from build123d import *

# Parameters (mm, degrees)
F0_R     = 36
F1_DEPTH = 125
F2_R     = 12.7
F3_DEPTH = 254
F4_R     = 10.16


with BuildPart() as f1:
    # F0 (on Right) → F1 (new body)
    with BuildSketch(Plane.YZ):
        with Locations((-19.977277, 22.49966)):
            Circle(F0_R)
    extrude(amount=F1_DEPTH)

    # F2 (on face) → F3 (cut)
    with BuildSketch(Plane(origin=(0, 0, 0), x_dir=(0, -1, 0), z_dir=(-1, 0, 0))):
        with Locations((19.977277, 22.49966)):
            Circle(F2_R)
    extrude(amount=-F3_DEPTH, mode=Mode.SUBTRACT)

    # F4
    f4_edges = [f1.edges().sort_by_distance(p)[0] for p in [
        (0, -55.977277, 22.49966),
        (125, -55.977277, 22.49966),
    ]]
    fillet(f4_edges, radius=F4_R)


solid = f1.part
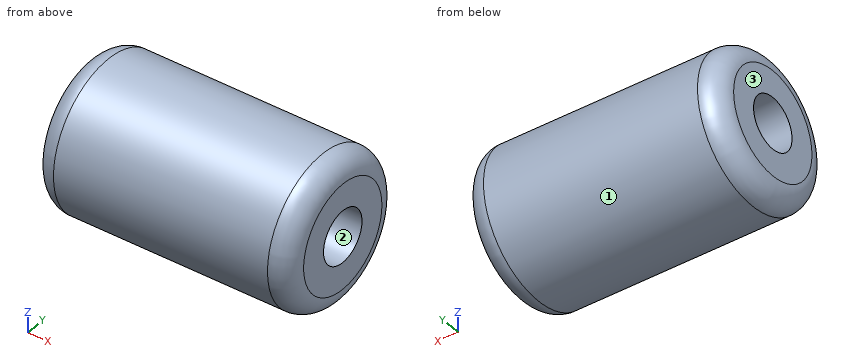
Geometry check sheet. Reference: the model listing, model coordinates, mm. Face numbers are marked on the shaded views. Round coordinates to 2 decimals unless told otherwise and drop trailing zeros. Order: outer loops, then holes, each group sorted by start corner. A loop starts at its lowest first (then second) coordinate and runs counter-clockwise, first axis right, second up. Notation, with made-up numbers: M -14,60.25 L 15,60.25 A34 ccw 15,95.25 Z; hole C 27,40.5 d9. An arc over 180 degrees is marked long. Answer in a Markdown table with one row per item.
(1) Sectioned sample at A-A, the plane x = 50. Record the cut outline in (y, z).
Responses:
| item | result |
|---|---|
| outline | C -19.98,22.5 d72; hole C -19.98,22.5 d25.4 |
(2) Go/stop test with flat-tipped pins: P1, Ø5, axis at x = 60, z = -5.5, coming from the -Y side; P2, Ø1, axis at x = 68, y = -7, coming from the +Z side; P3, Ø3, axis at x = 48, z = 18, coming from the +Y side. Record where each tip stops, or that it passes through.
Responses:
| item | result |
|---|---|
| P1 | stops at y = -45.39 |
| P2 | stops at z = 56.27 |
| P3 | stops at y = 15.9 |
(3) Scan lines: probe 1 along Z at (x, y) = (111.5, -20.5); probe 2 along Y at (x, z) = (31, 34); probe 3 along Y at (x, z) = (96.5, 20). Record each from-to range of solid material in increasing order. Write a range as from..to.
Responses:
| item | result |
|---|---|
| probe 1 | z = -13.5..9.81, 35.19..58.5 |
| probe 2 | y = -54.09..-25.37, -14.59..14.14 |
| probe 3 | y = -55.89..-32.43, -7.53..15.94 |
(4) Draft check along Z on the marked faces 1, 2 and 3. Enter one of: released by +Z, released by -Z, zero draft, split by the parting line, or undercut.
Responses:
| item | result |
|---|---|
| face 1 | split by the parting line |
| face 2 | undercut |
| face 3 | zero draft |
